```python
from build123d import *

# Parameters (mm, degrees)
SKIZZE1_W                       = 100
SKIZZE1_H                       = 5
AUFSATZ_LINEAR_AUSTRAGEN1_DEPTH = 5


with BuildPart() as part:
    # Skizze1 → Aufsatz-Linear austragen1 (new body)
    with BuildSketch(Plane.XY):
        with BuildLine():
            Line((97.5, -10), (102.5, -10))
            ThreePointArc((102.5, -10), (107.5, -15), (112.5, -10))
            Line((112.5, -10), (112.5, 10))
            Line((112.5, 10), (-112.5, 10))
            Line((-112.5, 10), (-112.5, -10))
            ThreePointArc((-112.5, -10), (-107.5, -15), (-102.5, -10))
            Line((-102.5, -10), (-97.5, -10))
            ThreePointArc((-97.5, -10), (-92.5, -15), (-87.5, -10))
            Line((-87.5, -10), (-52.5, -10))
            Line((-52.5, -10), (-47.5, -10))
            ThreePointArc((-47.5, -10), (-42.5, -15), (-37.5, -10))
            Line((-37.5, -10), (-12.5, -10))
            ThreePointArc((-12.5, -10), (-7.5, -15), (-2.5, -10))
            Line((-2.5, -10), (2.5, -10))
            ThreePointArc((2.5, -10), (7.5, -15), (12.5, -10))
            Line((12.5, -10), (37.5, -10))
            ThreePointArc((37.5, -10), (42.5, -15), (47.5, -10))
            Line((47.5, -10), (52.5, -10))
            ThreePointArc((52.5, -10), (57.5, -15), (62.5, -10))
            Line((62.5, -10), (87.5, -10))
            ThreePointArc((87.5, -10), (92.5, -15), (97.5, -10))
        make_face()
        with Locations((32.5, 12.5)):
            Rectangle(SKIZZE1_W, SKIZZE1_H)
        with BuildLine():
            Line((-52.5, -10), (-62.5, -10))
            ThreePointArc((-62.5, -10), (-57.5, -15), (-52.5, -10))
        make_face()
    extrude(amount=AUFSATZ_LINEAR_AUSTRAGEN1_DEPTH)


solid = part.part
```
Input: part model. Units: mm. Frame: model coordinates. A direction names the side the tool comes from. Give positions to 0.01 mm unless a question says otherwise; leave off trailing zeros. Order: outer loops, then holes, each group sorted by start corner. A loop starts at its lowest first (then second) coordinate and runs counter-clockwise, first axis right, second up. Notation, with made-up numbers: (37.25, 64.5) -> (68.25, 64.5) arc R23 ccw to (68.25, 85.5) -> close; hole circle Ø11 at (74, 16.25). An arc over 180 degrees is marked (long way). Write each question's results on one line, items separated by ' | '. Start each with the question number.
Item 1: Cut plane B-B on y = -12.5. Give the number of separate pieces and of enclosed holes in the cut face, then the cut area to 3 significant figures.
Item 2: Line query: line 1 (X direction, y = 12.75, z = 1.45); line 2 (Y direction, x = -1, z = 2.85); line 3 (Y direction, x = -50, z = 0.8). Output: solid intervals per line, ascending.
Item 3: Set-up query: faces 1 (the flat face through (-2, 0, 0)), 2 (the flat face through (98, 10, 2)), 3 (the flat face through (75, -10, 2)). Return all of +Z, -Z, +X, -X, +Y, -Y with unobstructed straight access to the full face (end or side cutting, diameter ignored); none if empty.
Item 4: Cut plane A-A on z = 1.95. Return the cut outline in (x, y), then the cut area to 3 significant figures.
Item 5: Mould query, pull axis X, two halves, no side actions, for faces 4 (the flat face through (-50, -10, 2)), 5 (the flat face through (0, -10, 2)), 6 (the flat face through (-112.5, 0, 2)), 7 (the flat face through (-64, 10, 2)). Classes: pulls with the +X half, pulls with the -X half, needs draft (parallel to the pull), parting line crosses it, or undercut.
Item 6: Contact query for a flat-ended pin moving along its axis: P1, Ø3, axis at x = 30, z = 3.5, coming from the -Y side. Output: stop coordinate, or through.
Item 7: Cut plane C-C on x = -92.5. Return the cut outline in (y, z), then the cut area to 3 significant figures.
Established:
1) separate pieces: 10 | enclosed holes: 0 | area: 433 mm^2
2) line 1: -17.5 to 82.5 | line 2: -10 to 15 | line 3: -10 to 10
3) face 1: -Z, +X, -X, +Y, -Y | face 2: +Z, -Z, +X, +Y | face 3: +Z, -Z, -Y
4) outline: (-112.5, -10) arc R5 ccw to (-102.5, -10) -> (-97.5, -10) arc R5 ccw to (-87.5, -10) -> (-62.5, -10) arc R5 ccw to (-52.5, -10) -> (-47.5, -10) arc R5 ccw to (-37.5, -10) -> (-12.5, -10) arc R5 ccw to (-2.5, -10) -> (2.5, -10) arc R5 ccw to (12.5, -10) -> (37.5, -10) arc R5 ccw to (47.5, -10) -> (52.5, -10) arc R5 ccw to (62.5, -10) -> (87.5, -10) arc R5 ccw to (97.5, -10) -> (102.5, -10) arc R5 ccw to (112.5, -10) -> (112.5, 10) -> (82.5, 10) -> (82.5, 15) -> (-17.5, 15) -> (-17.5, 10) -> (-112.5, 10) -> close | area: 5,390 mm^2
5) face 4: undercut | face 5: undercut | face 6: pulls with the -X half | face 7: needs draft
6) P1: y = -10
7) outline: (-15, 0) -> (10, 0) -> (10, 5) -> (-15, 5) -> close | area: 125 mm^2
